```python
from build123d import *

# Parameters (mm, degrees)
SKETCH1_W           = 76.2
SKETCH1_H           = 25.4
SKETCH1_W_2         = 70.104
SKETCH1_H_2         = 19.304
BOSS_EXTRUDE1_DEPTH = 241.091915
SKETCH3_W           = 76.2
SKETCH3_H           = 25.4
SKETCH3_W_2         = 70.104
SKETCH3_H_2         = 19.304
BOSS_EXTRUDE2_DEPTH = 3.048
SKETCH4_W           = 76.2
SKETCH4_H           = 25.4
SKETCH4_W_2         = 70.104
SKETCH4_H_2         = 19.304
BOSS_EXTRUDE3_DEPTH = 38.1
CUT_EXTRUDE2_START  = 105.580594
SKETCH5_R           = 38.1
CUT_EXTRUDE2_DEPTH  = 111.6566


with BuildPart() as part:
    # Sketch1 → Boss-Extrude1 (new body)
    with BuildSketch(Plane(origin=(0, 0, 0), x_dir=(1, 0, 0), z_dir=(0, 1, 0))):
        Rectangle(SKETCH1_W, SKETCH1_H)
        Rectangle(SKETCH1_W_2, SKETCH1_H_2, mode=Mode.SUBTRACT)
    extrude(amount=BOSS_EXTRUDE1_DEPTH)

    # Sketch3 → Boss-Extrude2 (add)
    with BuildSketch(Plane(origin=(0, 241.09191526, 0), x_dir=(1, 0, 0), z_dir=(0, 1, 0))):
        Rectangle(SKETCH3_W, SKETCH3_H)
        Rectangle(SKETCH3_W_2, SKETCH3_H_2, mode=Mode.SUBTRACT)
    extrude(amount=BOSS_EXTRUDE2_DEPTH)

    # Sketch4 → Boss-Extrude3 (add)
    with BuildSketch(Plane.XZ):
        Rectangle(SKETCH4_W, SKETCH4_H)
        Rectangle(SKETCH4_W_2, SKETCH4_H_2, mode=Mode.SUBTRACT)
    extrude(amount=BOSS_EXTRUDE3_DEPTH)

    # Sketch5 → Cut-Extrude2 (cut)
    with BuildSketch(Plane(origin=(-107.386524849, 327.150922863, -6.145385199), x_dir=(0.03097261, -0.032688156, -0.998985576), z_dir=(0.779560672, -0.624735905, 0.044611748)).offset(CUT_EXTRUDE2_START)):
        Circle(SKETCH5_R)
    extrude(amount=CUT_EXTRUDE2_DEPTH, mode=Mode.SUBTRACT)


solid = part.part
```
The model under review builds one solid part; all positions refer to its coordinate system, in mm. A direction names the side the tool comes from. Round coordinates to 2 decimals unless told otherwise and drop trailing zeros. Order: outer loops, then holes, each group sorted by start corner. A loop starts at its lowest first (then second) coordinate and runs counter-clockwise, first axis right, second up. Notation, with made-up numbers: (6.25, -23.75) - (12.25, -23.75) arc R22 ccw to (12.25, 11.25) - close; hole circle Ø9 at (75.25, 48.25). An arc over 180 degrees is marked (long way). Answer in a Markdown table with one row per item.
(1) Machinability: for faces 1 (the face through (-3, 196, 10)), 2 (the face through (0, 94, 9.652)), which of the approach directions +Z, -Z, +X, -X, +Y, -Y give a long, thin tool a straight path to every point of the face, cutting with its end or side? Answer none if there is none.
Result set:
| item | result |
|---|---|
| face 1 | +X, +Y |
| face 2 | +Y, -Y |
(2) Clearance check with a flat-ended pin moving along its axis: P1, Ø1, axis at y = 187, z = -1.5, coming from the +X side. State where the tip first meets the part, or that it passes through.
Result set:
| item | result |
|---|---|
| P1 | stops at x = -35.05 |
(3) Take a section at A-A on y = 22.5. Write out the cut boundary in (x, z).
Result set:
| item | result |
|---|---|
| outline | (-38.1, -12.7) - (38.1, -12.7) - (38.1, 12.7) - (-38.1, 12.7) - close; hole (-35.05, -9.65) - (35.05, -9.65) - (35.05, 9.65) - (-35.05, 9.65) - close |
(4) For line 1 (X direction, y = 91.5, z = 9.25); line 2 (Z direction, x = -14, y = 189); line 3 (X direction, y = 213.5, z = -4.25), list the stretches that pass through material, from the lowest coordinate up. Write a range as from..to.
Result set:
| item | result |
|---|---|
| line 1 | x = -38.1..-35.05, 35.05..38.1 |
| line 2 | z = -12.7..-9.65, 9.65..12.7 |
| line 3 | x = -38.1..-35.05 |
(5) Mouldability with a two-part tool opening along Z and no side actions: class faces 3 (the face through (-38.1, 96, 0)), 4 (the face through (-35.052, 94, 0)), 5 (the face through (-1, 66, -12.7)) as released by +Z, released by -Z, zero draft, split by the parting line, or undercut.
Result set:
| item | result |
|---|---|
| face 3 | zero draft |
| face 4 | undercut |
| face 5 | released by -Z |
